Geometry check sheet. Reference: the model listing, model coordinates, mm. Face numbers are marked on the shaded views. A direction names the side the tool comes from. Coordinates: 2 decimals unless noted, no trailing zeros. Loops run counter-clockwise (first coordinate to the right, second up) from the corner with the lowest first, then second, coordinate; pieces in that order, holes last. Notation, with made-up numbers: (-31, 68.25) - (-23, 68.25) arc R27 cw to (-23, 98.25) - close; hole circle Ø11 at (43.25, -4). An arc over 180 degrees is marked (long way). One line per item, written item: value.
from build123d import *

# Parameters (mm, degrees)
SKETCH007_W           = 10
SKETCH007_H           = 85.035517
EXTRUDE007_DEPTH      = 50
SKETCH006_R           = 7.5
EXTRUDE006_DEPTH      = 20
CLONE_PLACEMENT_ANGLE = 180


with BuildPart() as extrude007:
    # Sketch007 → Extrude007 (new body)
    with BuildSketch(Plane.XZ.offset(20)):
        with Locations((0, 17.482242)):
            Rectangle(SKETCH007_W, SKETCH007_H)
    extrude(amount=-EXTRUDE007_DEPTH)


with BuildPart() as cut003:
    # Sketch006 → Extrude006 (new body, symmetric)
    with BuildSketch(Plane.YZ):
        with BuildLine():
            ThreePointArc((-20, 9e-06), (1.3e-05, -20), (20, 3.6e-05))
            Line((20, 80), (20, 3.6e-05))
            Line((-20, 80), (20, 80))
            Line((-20, 9e-06), (-20, 80))
        make_face()
        Circle(SKETCH006_R, mode=Mode.SUBTRACT)
    extrude(amount=EXTRUDE006_DEPTH, both=True)

    # Cut002: cut Extrude007
    add(extrude007.part, mode=Mode.SUBTRACT)


with BuildPart() as cut003_1:
    # Clone placement: moved
    add(cut003.part.moved(Location((0, 0, 850))).rotate(Axis((0, 0, 850), (0, 1, 0)), CLONE_PLACEMENT_ANGLE))


solid = cut003_1.part
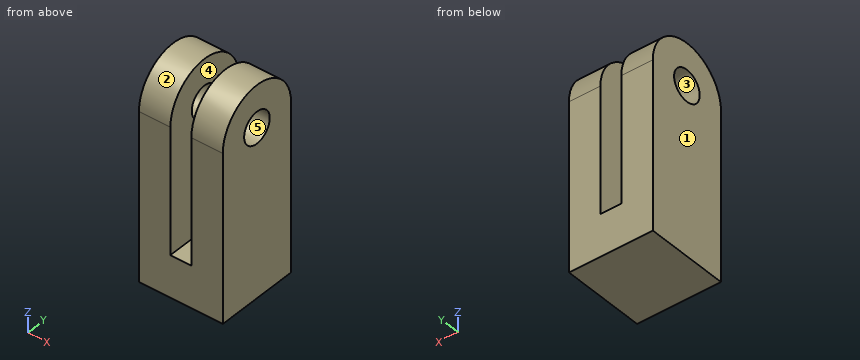
(1) Go/stop test with flat-tipped pins: pin 1 Ø5 at (x, y) = (-2, -4) entering from +Z; pin 2 Ø4 at (x, y) = (13.5, 8) entering from +Z; pin 3 Ø8 at (x, y) = (5, -1.5) entering from +Z; pin 4 Ø19.5 at (y, z) = (0, 850) entering from -X. Record where each tip stops, or that it passes through.
Reply:
pin 1: z = 790
pin 2: z = 869.08
pin 3: z = 870
pin 4: x = -20
(2) Material ranges on probe 1 along X at (y, z) = (-6, 860); probe 2 along Z at (x, y) = (-11, 0); probe 3 along Y at (x, z) = (14, 850), recorded low to high. Write a range as from..to.
Reply:
probe 1: -20..-5, 5..20
probe 2: 770..842.5, 857.5..870
probe 3: -20..-7.5, 7.5..20
(3) Cross-section at A-A on y = 0. Record the cut outline in (x, z), and give its area (3 significant figures).
Reply:
outline: (-20, 770) - (20, 770) - (20, 842.5) - (5, 842.5) - (5, 790) - (-5, 790) - (-5, 842.5) - (-20, 842.5) - close; (-20, 857.5) - (-5, 857.5) - (-5, 870) - (-20, 870) - close; (5, 857.5) - (20, 857.5) - (20, 870) - (5, 870) - close
area: 2,750 mm2
(4) Cross-section at B-B on z = 798. Record the cut outline in (x, y), and give its area (3 significant figures).
Reply:
outline: (-20, -20) - (-5, -20) - (-5, 20) - (-20, 20) - close; (5, -20) - (20, -20) - (20, 20) - (5, 20) - close
area: 1,200 mm2
(5) Access from +Z, -Z, +X, -X, +Y, -Y to the whole of each face (thin tool, end or side, straight path). Record for the marked faces 4 and 5.
Reply:
face 4: +Z, +Y, -Y
face 5: +X, -X
(6) Cross-section at D-D on z = 855.5. Record the cut outline in (x, y), and give its area (3 significant figures).
Reply:
outline: (-20, -19.23) - (-5, -19.23) - (-5, -5.1) - (-20, -5.1) - close; (-20, 5.1) - (-5, 5.1) - (-5, 19.23) - (-20, 19.23) - close; (5, -19.23) - (20, -19.23) - (20, -5.1) - (5, -5.1) - close; (5, 5.1) - (20, 5.1) - (20, 19.23) - (5, 19.23) - close
area: 848 mm2
(7) Cross-section at C-C on x = 6.5. Record the cut outline in (y, z).
Reply:
outline: (-20, 770) - (20, 770) - (20, 850) arc R20 ccw to (-20, 850) - close; hole circle Ø15 at (0, 850)
(8) Release check for a two-part mould opening along Z. For the marked faces 1, 2 and 3 record: pulls with the +Z half, pulls with the -Z half, needs draft (parallel to the pull), parting line crosses it, or undercut.
Reply:
face 1: needs draft
face 2: pulls with the +Z half
face 3: undercut
